```python
from build123d import *

# Parameters (mm, degrees)
ESBO_O1_W                = 7.305190172
ESBO_O1_H                = 2.5
ESBO_O1_H_2              = 3
RESSALTO_EXTRUS_O1_DEPTH = 4
CUT_EXTRUDE1_DEPTH       = 10
FURO_COM_FOLGA_DE_M31_D  = 3.2
FILLET1_R                = 3


with BuildPart() as part:
    # Esboço1 → Ressalto-extrusão1 (new body)
    with BuildSketch(Plane.XY):
        with BuildLine():
            Line((-49.295269139, -236.354481491), (30.295730877, -236.354481491))
            ThreePointArc((30.295730877, -236.354481491), (32.417051221, -237.233161147), (33.295730877, -239.354481491))
            Line((33.295730877, -239.354481491), (33.295730877, -245.447951064))
            ThreePointArc((33.295730877, -245.447951064), (34.174410534, -247.569271408), (36.295730877, -248.447951064))
            Line((36.295730877, -248.447951064), (46.077297056, -248.447951064))
            ThreePointArc((46.077297056, -248.447951064), (48.198617399, -247.569271408), (49.077297056, -245.447951064))
            Line((49.077297056, -245.447951064), (49.077297056, -239.354481491))
            ThreePointArc((49.077297056, -239.354481491), (49.955976712, -237.233161147), (52.077297056, -236.354481491))
            Line((52.077297056, -236.354481491), (68.643919436, -236.354481491))
            ThreePointArc((68.643919436, -236.354481491), (70.765239779, -235.475801834), (71.643919436, -233.354481491))
            Line((71.643919436, -233.354481491), (71.643919436, -231.207792375))
            Line((71.643919436, -231.207792375), (84.613919436, -231.207792375))
            Line((84.613919436, -231.207792375), (84.613919436, -65.265257908))
            Line((84.613919436, -65.265257908), (71.643919436, -65.265257908))
            Line((71.643919436, -65.265257908), (71.643919436, -47.354481491))
            ThreePointArc((71.643919436, -47.354481491), (70.765239779, -45.233161147), (68.643919436, -44.354481491))
            Line((68.643919436, -44.354481491), (-79.423286283, -44.354481491))
            ThreePointArc((-79.423286283, -44.354481491), (-81.544606627, -45.233161147), (-82.423286283, -47.354481491))
            Line((-82.423286283, -47.354481491), (-82.423286283, -65.265257908))
            Line((-82.423286283, -65.265257908), (-99.449266915, -65.265257908))
            Line((-99.449266915, -65.265257908), (-99.449266915, -233.354481491))
            ThreePointArc((-99.449266915, -233.354481491), (-98.570587259, -235.475801834), (-96.449266915, -236.354481491))
            Line((-96.449266915, -236.354481491), (-68.333570548, -236.354481491))
            ThreePointArc((-68.333570548, -236.354481491), (-66.212250205, -237.233161147), (-65.333570548, -239.354481491))
            Line((-65.333570548, -239.354481491), (-65.333570548, -240.354481491))
            ThreePointArc((-65.333570548, -240.354481491), (-64.454890892, -242.475801834), (-62.333570548, -243.354481491))
            Line((-62.333570548, -243.354481491), (-55.295269139, -243.354481491))
            ThreePointArc((-55.295269139, -243.354481491), (-53.173948795, -242.475801834), (-52.295269139, -240.354481491))
            Line((-52.295269139, -240.354481491), (-52.295269139, -239.354481491))
            ThreePointArc((-52.295269139, -239.354481491), (-51.416589482, -237.233161147), (-49.295269139, -236.354481491))
        make_face()
        with Locations((40.863663265, -239.358820259)):
            Rectangle(ESBO_O1_W, ESBO_O1_H, mode=Mode.SUBTRACT)
        with Locations((40.863663265, -243.481650875)):
            Rectangle(ESBO_O1_W, ESBO_O1_H_2, mode=Mode.SUBTRACT)
        with Locations((40.863663265, -51.350142723)):
            Rectangle(ESBO_O1_W, ESBO_O1_H, mode=Mode.SUBTRACT)
        with Locations((40.863663265, -47.227312107)):
            Rectangle(ESBO_O1_W, ESBO_O1_H_2, mode=Mode.SUBTRACT)
    extrude(amount=RESSALTO_EXTRUS_O1_DEPTH)

    # Sketch1 → Cut-Extrude1 (cut)
    with BuildSketch(Plane.XY.offset(4)):
        with BuildLine():
            Line((-79.386080564, -236.354481491), (-79.386080564, -228.792861815))
            Line((-79.386080564, -228.792861815), (-79.386080564, -205.765971774))
            Line((-79.386080564, -205.765971774), (-70.386080564, -205.765971774))
            Line((-70.386080564, -205.765971774), (-70.386080564, -225.792861815))
            Line((-70.386080564, -225.792861815), (59.613919436, -225.792861815))
            Line((59.613919436, -225.792861815), (59.613919436, -205.765971774))
            Line((59.613919436, -205.765971774), (68.613919436, -205.765971774))
            Line((68.613919436, -205.765971774), (68.613919436, -228.792861815))
            Line((68.613919436, -228.792861815), (68.613919436, -236.354481491))
            Line((68.613919436, -236.354481491), (68.643919436, -236.354481491))
            ThreePointArc((68.643919436, -236.354481491), (70.765239779, -235.475801834), (71.643919436, -233.354481491))
            Line((71.643919436, -233.354481491), (71.643919436, -231.207792375))
            Line((71.643919436, -231.207792375), (84.613919436, -231.207792375))
            Line((84.613919436, -231.207792375), (84.613919436, -65.265257908))
            Line((84.613919436, -65.265257908), (71.643919436, -65.265257908))
            Line((71.643919436, -65.265257908), (71.643919436, -47.354481491))
            ThreePointArc((71.643919436, -47.354481491), (70.765239779, -45.233161147), (68.643919436, -44.354481491))
            Line((68.643919436, -44.354481491), (-79.423286283, -44.354481491))
            ThreePointArc((-79.423286283, -44.354481491), (-81.544606627, -45.233161147), (-82.423286283, -47.354481491))
            Line((-82.423286283, -47.354481491), (-82.423286283, -65.265257908))
            Line((-82.423286283, -65.265257908), (-99.449266915, -65.265257908))
            Line((-99.449266915, -65.265257908), (-99.449266915, -233.354481491))
            ThreePointArc((-99.449266915, -233.354481491), (-98.570587259, -235.475801834), (-96.449266915, -236.354481491))
            Line((-96.449266915, -236.354481491), (-79.386080564, -236.354481491))
        make_face()
    extrude(amount=-CUT_EXTRUDE1_DEPTH, mode=Mode.SUBTRACT)

    # Furo com folga de M31 (through all)
    with Locations(Plane.XY.offset(4)):
        with Locations((-74.886080564, -50.354481491), (64.113919436, -230.354481491), (64.113919436, -50.354481491), (-74.886080564, -230.354481491), (-59.12185492, -47.477548601), (-5.386080564, -50.354481491), (-59.12185492, -238.651414381), (-5.386080564, -230.354481491), (64.113919436, -210.354481491), (-74.886080564, -210.354481491)):
            Hole(FURO_COM_FOLGA_DE_M31_D / 2)

    # Fillet1
    fillet1_edges = [part.edges().sort_by_distance(p)[0] for p in [
        (-79.386080564, -236.354481491, 2),
        (68.613919436, -205.765971774, 2),
        (59.613919436, -205.765971774, 2),
        (59.613919436, -225.792861815, 2),
        (-70.386080564, -225.792861815, 2),
        (-70.386080564, -205.765971774, 2),
        (-79.386080564, -205.765971774, 2),
        (68.613919436, -236.354481491, 2),
    ]]
    fillet(fillet1_edges, radius=FILLET1_R)


solid = part.part
```
The listing builds one solid part. Answer for the finished solid, in the listing's coordinates (mm). A direction names the side the tool comes from. Coordinates: 2 decimals unless noted, no trailing zeros. Write each loop counter-clockwise with the first axis right and the second up, starting at its lowest first coordinate (ties: lowest second). Pieces come first, ordered by that corner, then holes.
Q1. The mould has two halves that part along X. Classify faces 1 (the flat face through (41, -244.982, 2)), 2 (the cylindrical face through (67.76, -206.67, 1.97)), 3 (the cylindrical face through (-78.484, -235.499, 1.972)): released by +X, released by -X, zero draft, split by the parting line, or undercut.
Returned:
face 1: undercut
face 2: released by +X
face 3: released by -X
Q2. Section A-A, the plane y = -220 is taken. Write down the section's boundary in (x, z).
Returned:
outline: (-79.39, 0) - (-70.39, 0) - (-70.39, 4) - (-79.39, 4) - close; (59.61, 0) - (68.61, 0) - (68.61, 4) - (59.61, 4) - close
Q3. Section B-B, the plane x = 23 is taken. Write down the section's boundary in (y, z).
Returned:
outline: (-236.35, 0) - (-225.79, 0) - (-225.79, 4) - (-236.35, 4) - close
Q4. Find the intervals of material crossed by line 1 along Y through (x, z) = (43, 1.25); line 2 along X through (y, z) = (-244.5, 1.65); line 3 along X through (y, z) = (-218, 2.7), in increasing order.
Returned:
line 1: y = -248.45 to -244.98, -241.98 to -240.61, -238.11 to -225.79
line 2: x = 33.3 to 37.21, 44.52 to 49.08
line 3: x = -79.39 to -70.39, 59.61 to 68.61
Q5. Which of the six approach directions +Z, -Z, +X, -X, +Y, -Y give full straight-line access (tool end or side, diameter ignored) to faces 4 (the cylindrical face through (-53.2, -242.5, 2)), 5 (the flat face through (37.211, -244, 2)), 6 (the cylindrical face through (-69.53, -224.89, 1.97))?
Returned:
face 4: +Z, -Z, -Y
face 5: +Z, -Z
face 6: +Z, -Z, +Y
Q6. Given P1, Ø0.8, axis at y = -239.5, z = 1, coming from the -X side; P2, Ø2, axis at x = 7.5, z = 2.5, coming from the -Y side; P3, Ø0.9, axis at y = -244, z = 2.5, coming from the +X side, each flat-ended and moving along its own axis, determine where each tip first touches the part or whether it passes through.
Returned:
P1: stops at x = -65.34
P2: stops at y = -236.35
P3: stops at x = 49.08
Q7. Section C-C, the plane z = 2.8 is taken. Give the number of separate pieces and of enclosed holes in the cut face, then the cut area to 3 significant figures.
Returned:
separate pieces: 1
enclosed holes: 8
area: 2,110 mm2
